Here's how the part is built. I have some questions about the finished solid (model axes, mm). A direction names the side the tool comes from. Round coordinates to 2 decimals unless told otherwise and drop trailing zeros. Write each loop counter-clockwise with the first axis right and the second up, starting at its lowest first coordinate (ties: lowest second). Pieces come first, ordered by that corner, then holes. Notation, with made-up numbers: (56.5, 66.25) - (63.5, 66.25) arc R17 ccw to (63.5, 89.25) - close; hole circle Ø9 at (-32, 77). An arc over 180 degrees is marked (long way). Use one line per item in the form item = value. Start each with the question number.
1. We'd pull the mould along Y, two halves only. Please class faces 4 (the cylindrical face through (18.11, -17.57, 12.52)), 5 (the flat face through (-22, 38.1, 13)), 6 (the flat face through (4.445, 29, 13)): +Y half, -Y half, draft (parallel to the pull), parting line (faces both ways), or undercut.
2. I want a section at B-B, the plane y = 19.05. List the corners of the cut face in (x, z) for me (3 decimals), plus the area to 3 significant figures.
3. Which directions (+Z, -Z, +X, -X, +Y, -Y) give clear straight access to the entire face, cutting with the end or side of a thin tool? Please do faces 1 (the flat face through (16, 1, 0)), 2 (the flat face through (-9.525, 0, 13)), 3 (the flat face through (-4.445, 29, 13)).
4. I want a section at C-C, the plane y = -14.5. List the corners of the cut face in (x, z) for me (3 decimals), plus the area to 3 significant figures.
5. Will this pin go through, and if not, where does the flat tip stop? pin 1 (2 mm diameter, centred on x = 19.05, y = -19.05, fed in from -Z).
6. I want a section at D-D, the plane z = 5. State how many separate pieces and enclosed holes the cut face has, plus the area to 3 significant figures.
7. I want a section at A-A, the plane x = -19.05. List the corners of the cut face in (y, z) for me, plus the area to 3 significant figures.
8. If I drill on line 1 along Y through (x, z) = (-19.05, 10.25); line 2 along Y through (x, z) = (6, 9); line 3 along X through (y, z) = (-17, 4.75) (3 decimals), over which ranges is the centre line in solid material (lowest first)?
```python
from build123d import *

# Parameters (mm, degrees)
F0_W     = 76.2
F0_H     = 76.2
F1_DEPTH = 25.4
F2_W     = 19.05
F2_H     = 41.275
F3_DEPTH = 25.4
F4_W     = 8.89
F4_H     = 17.4625
F5_DEPTH = 25.4
F7_D     = 3.5052


with BuildPart() as f1:
    # F0 (on Top) → F1 (new body)
    with BuildSketch(Plane.XY):
        Rectangle(F0_W, F0_H)
    extrude(amount=F1_DEPTH)

    # F2 (on face) → F3 (cut)
    with BuildSketch(Plane.XY.offset(25.4)):
        Rectangle(F2_W, F2_H)
    extrude(amount=-F3_DEPTH, mode=Mode.SUBTRACT)

    # F4 (on face) → F5 (cut)
    with BuildSketch(Plane.XY.offset(25.4)):
        with Locations((0, 29.36875)):
            Rectangle(F4_W, F4_H)
    extrude(amount=-F5_DEPTH, mode=Mode.SUBTRACT)

    # F7 (through all)
    with Locations(Plane.XY.offset(25.4)):
        with Locations((-19.05, 19.05), (-19.05, -19.05), (19.05, -19.05), (19.05, 19.05)):
            Hole(F7_D / 2)


solid = f1.part
```
Model answer:
q1.face_4 = undercut
q1.face_5 = +Y half
q1.face_6 = draft
q2.outline = (-38.1, 0) - (-20.803, 0) - (-20.803, 25.4) - (-38.1, 25.4) - close; (-17.297, 0) - (-9.525, 0) - (-9.525, 25.4) - (-17.297, 25.4) - close; (9.525, 0) - (17.297, 0) - (17.297, 25.4) - (9.525, 25.4) - close; (20.803, 0) - (38.1, 0) - (38.1, 25.4) - (20.803, 25.4) - close
q2.area = 1,270 mm2
q3.face_1 = -Z, +X, -X, +Y, -Y
q3.face_2 = +Z, -Z
q3.face_3 = +Z, -Z, +Y
q4.outline = (-38.1, 0) - (-9.525, 0) - (-9.525, 25.4) - (-38.1, 25.4) - close; (9.525, 0) - (38.1, 0) - (38.1, 25.4) - (9.525, 25.4) - close
q4.area = 1,450 mm2
q5.pin_1 = through
q6.separate_pieces = 1
q6.enclosed_holes = 4
q6.area = 4,830 mm2
q7.outline = (-38.1, 0) - (-20.8, 0) - (-20.8, 25.4) - (-38.1, 25.4) - close; (-17.3, 0) - (17.3, 0) - (17.3, 25.4) - (-17.3, 25.4) - close; (20.8, 0) - (38.1, 0) - (38.1, 25.4) - (20.8, 25.4) - close
q7.area = 1,760 mm2
q8.line_1 = -38.1 to -20.8, -17.3 to 17.3, 20.8 to 38.1
q8.line_2 = -38.1 to -20.64, 20.64 to 38.1
q8.line_3 = -38.1 to -9.525, 9.525 to 38.1
